Input: dimensioned drawing with shaded views. Units: mm. Origin: part minimum x, y, z. A direction names the side the tool comes from. Coordinates: 2 decimals unless noted, no trailing zeros. Loops run counter-clockwise (first coordinate to the right, second up) from the corner with the lowest first, then second, coordinate; pieces in that order, holes last.
(1) Set-up query: the marked faces 1 and 2. Return all of +Z, -Z, +X, -X, +Y, -Y with unobstructed straight access to the full face (end or side cutting, diameter ignored); none if empty.
(2) Section A-A, the plane z = 14. Return loops of the section in (x, y).
(3) Section B-B, the plane x = 5.75. Return loops of the section in (y, z).
(4) Mould query, pull axis Z, two halves, no side actions, for the marked faces 3, 4 and 5. Classes: released by +Z, released by -Z, zero draft, split by the parting line, or undercut.
(5) Line query: L1, parallel to X at y = 1.75, z = 7.75; L2, parallel to Z at x = 7, y = 1.8. Output: solid intervals per line, ascending.
(6) Section C-C, the plane y = 3.9. Return loops of the section in (x, z), then the cut area to 3 significant figures.
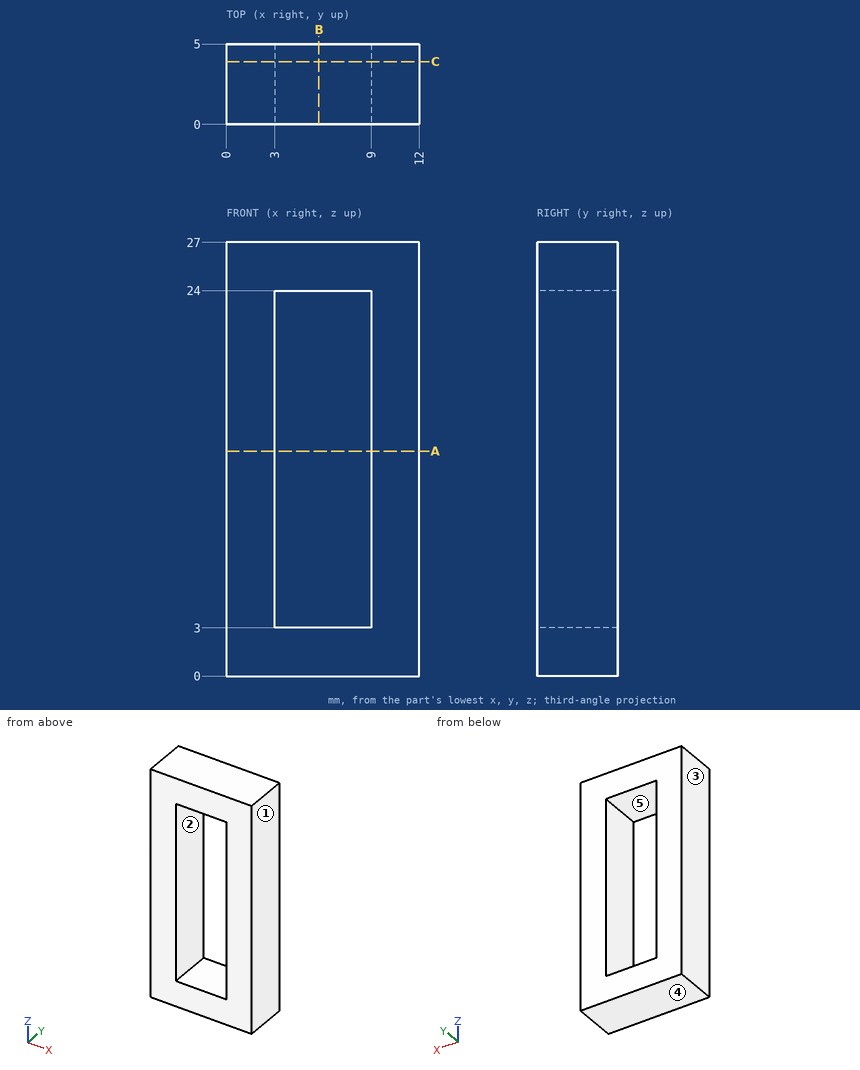
Report:
1. face 1: +Z, -Z, +X, +Y, -Y
1. face 2: +Y, -Y
2. outline: (0, 0) - (3, 0) - (3, 5) - (0, 5) - close; (9, 0) - (12, 0) - (12, 5) - (9, 5) - close
3. outline: (0, 0) - (5, 0) - (5, 3) - (0, 3) - close; (0, 24) - (5, 24) - (5, 27) - (0, 27) - close
4. face 3: zero draft
4. face 4: released by -Z
4. face 5: undercut
5. L1: x = 0 to 3, 9 to 12
5. L2: z = 0 to 3, 24 to 27
6. outline: (0, 0) - (12, 0) - (12, 27) - (0, 27) - close; hole (3, 3) - (9, 3) - (9, 24) - (3, 24) - close
6. area: 198 mm2
